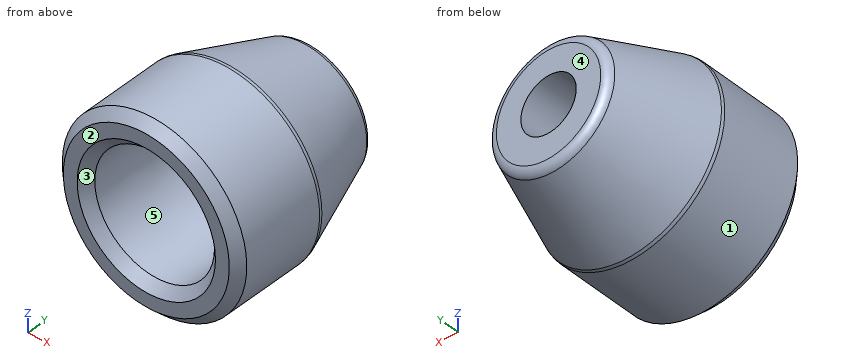
```python
from build123d import *
from OCP.BRepFilletAPI import BRepFilletAPI_MakeChamfer

# Parameters (mm, degrees)
SKETCH1_R           = 5
BOSS_EXTRUDE1_DEPTH = 10
SKETCH2_R           = 1.5
CUT_EXTRUDE1_DEPTH  = 13.247448714
CHAMFER1_SIZE       = 5
CHAMFER1_SIZE2      = 1.819851171
SKETCH3_R           = 3.25
CUT_EXTRUDE2_DEPTH  = 6.940927836
CUT_EXTRUDE2_DRAFT  = -0.5
CHAMFER2_SIZE       = 0.5
CHAMFER2_SIZE2      = 0.504421055
FILLET1_R           = 0.5


with BuildPart() as part:
    # Sketch1 → Boss-Extrude1 (new body)
    with BuildSketch(Plane(origin=(0, 0, 0), x_dir=(1, 0, 0), z_dir=(0, 1, 0))):
        with Locations(Location((0, 0, 0), (0, 0, 270))):
            Circle(SKETCH1_R)
    extrude(amount=BOSS_EXTRUDE1_DEPTH)

    # Sketch2 → Cut-Extrude1 (cut, through all)
    with BuildSketch(Plane(origin=(0, 10, 0), x_dir=(1, 0, 0), z_dir=(0, 1, 0))):
        with Locations(Location((0, 0, 0), (0, 0, 270))):
            Circle(SKETCH2_R)
    extrude(amount=-CUT_EXTRUDE1_DEPTH, mode=Mode.SUBTRACT)

    # Chamfer1
    chamfer1_edges = [part.edges().sort_by_distance(p)[0] for p in [
        (0, 10, -5),
    ]]
    chamfer1_side = [part.faces().sort_by_distance(p)[0] for p in [
        (0, 5, -5),
    ]]
    chamfer(chamfer1_edges, length=CHAMFER1_SIZE, length2=CHAMFER1_SIZE2, reference=chamfer1_side[0])


with BuildPart() as cut_extrude2_tool:
    # Sketch3 → Cut-Extrude2 (with draft: the straight prism first)
    with BuildSketch(Plane.XZ):
        Circle(SKETCH3_R)
    extrude(amount=-CUT_EXTRUDE2_DEPTH)
    # Cut-Extrude2: the draft: its side faces are tilted about the plane it starts from
    cut_extrude2_sides = [cut_extrude2_tool.faces().sort_by_distance(p)[0] for p in [
        (-3.25, 3.470463918, 0),
    ]]
    draft(cut_extrude2_sides, Plane.XZ, CUT_EXTRUDE2_DRAFT)


with BuildPart() as part_1:
    add(part.part)

    # Cut-Extrude2: cut by cut_extrude2_tool
    add(cut_extrude2_tool.part, mode=Mode.SUBTRACT)

    # Chamfer2: one chamfer whose edges measure the first distance from different faces: ONE call of the kernel's chamfer builder (chamfer() names one face for all edges)
    chamfer2_edges_1 = [part_1.edges().sort_by_distance(p)[0] for p in [
        (-3.25, 0, 0),
    ]]
    chamfer2_side_1 = [part_1.faces().sort_by_distance(p)[0] for p in [
        (0, 0, -4.858578644),
    ]]
    chamfer2_edges_2 = [part_1.edges().sort_by_distance(p)[0] for p in [
        (0, 0, -5),
    ]]
    chamfer2 = BRepFilletAPI_MakeChamfer(part_1.part.solid().wrapped)
    for e in chamfer2_edges_1:
        chamfer2.Add(CHAMFER2_SIZE, CHAMFER2_SIZE2, e.wrapped, chamfer2_side_1[0].wrapped)  # the first distance lies on this face
    for e in chamfer2_edges_2:
        chamfer2.Add(CHAMFER2_SIZE, e.wrapped)
    add(Compound.cast(chamfer2.Shape()), mode=Mode.REPLACE)

    # Fillet1
    fillet1_edges = [part_1.edges().sort_by_distance(p)[0] for p in [
        (0, 5, -5),
        (0, 10, -3.180148829),
    ]]
    fillet(fillet1_edges, radius=FILLET1_R)


solid = part_1.part
```
Here's how the part is built. I have some questions about the finished solid (model axes, mm). Face numbers are marked on the shaded views. A direction names the side the tool comes from. Round coordinates to 2 decimals unless told otherwise and drop trailing zeros. Loops run counter-clockwise (first coordinate to the right, second up) from the corner with the lowest first, then second, coordinate; pieces in that order, holes last.
1. If I drill on probe 1 along Y at (x, z) = (-1, -1.25); probe 2 along Z at (x, y) = (-1.25, 8.75); probe 3 along X at (y, z) = (8.1, 0), over which ranges is the centre line in solid material (lowest first)?
Answers:
probe 1: y = 6.94 to 10
probe 2: z = -3.41 to -0.83, 0.83 to 3.41
probe 3: x = -3.87 to -1.5, 1.5 to 3.87
2. Thinking about a two-plate mould opening in X: for the marked faces 1, 2 and 3, which applies, released by +X, released by -X, zero draft, split by the parting line, or undercut?
Answers:
face 1: split by the parting line
face 2: zero draft
face 3: undercut
3. Will these pins go through, and if not, where does the flat tip stop? pin 1 (3 mm diameter, centred on x = 1.5, z = -0.5, fed in from -Y); pin 2 (4 mm diameter, centred on x = -1.5, z = 0.5, fed in from -Y); pin 3 (4 mm diameter, centred on y = 9, z = -1, fed in from +X); pin 4 (2.5 mm diameter, centred on x = 0, z = 0, fed in from +Y).
Answers:
pin 1: stops at y = 6.94
pin 2: stops at y = 0.17
pin 3: stops at x = 4.22
pin 4: passes through
4. For the marked faces 4 and 5, which set-ups out of +Z, -Z, +X, -X, +Y, -Y let a thin tool reach every point of the face, with its end or its side?
Answers:
face 4: +Z, -Z, +X, -X, +Y
face 5: -Y
5. Suppose I cut it at A-A, the plane y = 1. Please give me the cut outline in (x, z), and give its area (3 significant figures).
Answers:
outline: circle Ø10 at (0, 0); hole circle Ø6.48 at (0, 0)
area: 45.5 mm2
